Design review of the part built by this model. Coordinates are the model's own, in mm. A direction names the side the tool comes from. Round coordinates to 2 decimals unless told otherwise and drop trailing zeros. Loops run counter-clockwise (first coordinate to the right, second up) from the corner with the lowest first, then second, coordinate; pieces in that order, holes last. Notation, with made-up numbers: (-36.75, -37) - (-6.75, -37) arc R21 cw to (-6.75, -10) - close; hole circle Ø4 at (23.25, -12.75). An arc over 180 degrees is marked (long way). Use one line per item in the form item = value. Start each with the question number.
(1) Wall thickness on probe 1 along Y at (x, z) = (15.5, -20.5); probe 2 along Z at (x, y) = (15, 5.25); probe 3 along Z at (x, y) = (4.75, 1.25): over which ranges is each line inside the solid? List them lowest first. Write a range as [from, to].
(2) We need section D-D, the plane y = 3. Write out the cut boundary in (x, z).
(3) We need section B-B, the plane z = -26. Write out the cut boundary in (x, y), then the cut area to 3 significant figures.
(4) For pin 1 (1.8 mm diameter, centred on x = 9, y = 2, fed in from -Z); pin 2 (1.1 mm diameter, centred on x = 4, z = -27, fed in from +Y), all flat-tipped, find the tip position at first contact; note any pin that passes through.
(5) We need section A-A, the plane y = 1.5. Write out the cut boundary in (x, z), then the cut area to 3 significant figures.
(6) We need section C-C, the plane x = 12.25. Write out the cut boundary in (y, z), then the cut area to 3 significant figures.
(7) The part is to be moulded in two halves that separate along Y. For faces 1 (the flat face through (9, 0, -13)), 2 (the flat face through (18.44, 3, -13)), 3 (the flat face through (4, 3.5, -25)), say which applies: released by +Y, released by -Y, zero draft, split by the parting line, or undercut.
(8) Machinability: for faces 4 (the flat face through (4, 4, -25)), 5 (the flat face through (9, 3, -20)), 6 (the flat face through (4, 1, -32)), 7 (the flat face through (4, 1, -31.5)), which of the approach directions +Z, -Z, +X, -X, +Y, -Y give a long, thin tool a straight path to every point of the face, cutting with its end or side? Answer none if there is none.
from build123d import *

# Parameters (mm, degrees)
EXTRUDE1_DEPTH     = 25
FILLET1_R          = 0.5
SKETCH3_W          = 16.44
SKETCH3_H          = 4
CUT_EXTRUDE1_DEPTH = 5
PROFILE_W          = 1
PROFILE_H          = 0.5


with BuildPart() as part:
    # Sketch2 → Extrude1 (new body)
    with BuildSketch(Plane.XY):
        with BuildLine():
            Line((0.5, 0), (17.94, 0))
            ThreePointArc((17.94, 0), (18.293553391, 0.146446609), (18.44, 0.5))
            Line((18.44, 0.5), (18.44, 5.5))
            ThreePointArc((18.44, 5.5), (18.293553391, 5.853553391), (17.94, 6))
            Line((17.94, 6), (0.5, 6))
            ThreePointArc((0.5, 6), (0.146446609, 5.853553391), (0, 5.5))
            Line((0, 5.5), (0, 0.5))
            ThreePointArc((0, 0.5), (0.146446609, 0.146446609), (0.5, 0))
        make_face()
    extrude(amount=-EXTRUDE1_DEPTH)

    # Fillet1
    fillet1_edges = [part.edges().sort_by_distance(p)[0] for p in [
        (9.22, 6, 0),
        (18.293553391, 5.853553391, 0),
        (18.44, 3, 0),
        (18.293553391, 0.146446609, 0),
        (9.22, 0, 0),
        (0.146446609, 0.146446609, 0),
        (0, 3, 0),
        (0.146446609, 5.853553391, 0),
    ]]
    fillet(fillet1_edges, radius=FILLET1_R)

    # Sketch3 → Cut-Extrude1 (cut)
    with BuildSketch(Plane(origin=(0, 0, -25), x_dir=(-1, 0, 0), z_dir=(0, 0, -1))):
        with Locations((-9.22, 3)):
            Rectangle(SKETCH3_W, SKETCH3_H)
    extrude(amount=-CUT_EXTRUDE1_DEPTH, mode=Mode.SUBTRACT)

    # Sweep1: sweep along a path in Path
    with BuildLine(Plane(origin=(9.22, 0, 0), x_dir=(0, 0, -1), z_dir=(1, 0, 0))) as sweep1_path:
        Line((20, 3.5), (30, 3.5))
        ThreePointArc((30, 3.5), (31.060660172, 3.060660172), (31.5, 2))
        Line((31.5, 2), (31.5, 0))
    # Profile → Sweep1 (sweep)
    with BuildSketch(Plane(origin=(0, 0, -20), x_dir=(-1, 0, 0), z_dir=(0, 0, -1))):
        with Locations((-14.76, 3.75)):
            Rectangle(PROFILE_W, PROFILE_H)
        with Locations((-3.68, 3.75)):
            Rectangle(PROFILE_W, PROFILE_H)
    sweep(path=sweep1_path.line)


solid = part.part
Data:
q1.probe_1 = [0, 1], [5, 6]
q1.probe_2 = [-25, 0]
q1.probe_3 = [-20, 0]
q2.outline = (0, -25) - (1, -25) - (1, -20) - (17.44, -20) - (17.44, -25) - (18.44, -25) - (18.44, -0.5) arc R0.5 ccw to (17.94, 0) - (0.5, 0) arc R0.5 ccw to (0, -0.5) - close; (3.18, -31.73) - (4.18, -31.73) - (4.18, -31.12) - (3.18, -31.12) - close; (14.26, -31.73) - (15.26, -31.73) - (15.26, -31.12) - (14.26, -31.12) - close
q3.outline = (3.18, 3.5) - (4.18, 3.5) - (4.18, 4) - (3.18, 4) - close; (14.26, 3.5) - (15.26, 3.5) - (15.26, 4) - (14.26, 4) - close
q3.area = 1.00 mm^2
q4.pin_1 = -20
q4.pin_2 = 4
q5.outline = (0, -25) - (1, -25) - (1, -20) - (17.44, -20) - (17.44, -25) - (18.44, -25) - (18.44, -0.5) arc R0.5 ccw to (17.94, 0) - (0.5, 0) arc R0.5 ccw to (0, -0.5) - close; (3.18, -32) - (4.18, -32) - (4.18, -31.5) - (3.18, -31.5) - close; (14.26, -32) - (15.26, -32) - (15.26, -31.5) - (14.26, -31.5) - close
q5.area = 380 mm^2
q6.outline = (0, -25) - (1, -25) - (1, -20) - (5, -20) - (5, -25) - (6, -25) - (6, -0.5) arc R0.5 ccw to (5.5, 0) - (0.5, 0) arc R0.5 ccw to (0, -0.5) - close
q6.area = 130 mm^2
q7.face_1 = released by -Y
q7.face_2 = zero draft
q7.face_3 = undercut
q8.face_4 = -Z
q8.face_5 = none
q8.face_6 = -Z, +X, -X, +Y, -Y
q8.face_7 = +X, -X, -Y
